Verification items for the finished model (mm, model axes). Coordinates: 2 decimals unless noted, no trailing zeros. Order: outer loops, then holes, each group sorted by start corner. A loop starts at its lowest first (then second) coordinate and runs counter-clockwise, first axis right, second up. Notation, with made-up numbers: M 77,69 L 128,69 A13 cw 128,93 Z; hole C 10.5,53.25 d7. An arc over 180 degrees is marked long. Write item = value, one per line.
```python
from build123d import *

# Parameters (mm, degrees)
SKETCH1_W      = 9.525
SKETCH1_H      = 24.13
EXTRUDE1_DEPTH = 9.525
SKETCH2_R      = 1.5875
EXTRUDE2_DEPTH = 10.525
EXTRUDE3_DEPTH = 9.525


with BuildPart() as part:
    # Sketch1 → Extrude1 (new body)
    with BuildSketch(Plane(origin=(0, 0, 0), x_dir=(1, 0, 0), z_dir=(0, 1, 0))):
        Rectangle(SKETCH1_W, SKETCH1_H)
    extrude(amount=EXTRUDE1_DEPTH)

    # Sketch2 → Extrude2 (cut, through all)
    with BuildSketch(Plane(origin=(4.7625, 0, 0), x_dir=(0, 0, -1), z_dir=(1, 0, 0))):
        with Locations((-6.35, 4.7625)):
            Circle(SKETCH2_R)
        with Locations(Location((6.35, 4.7625, 0), (0, 0, 180))):  # turned: the seam where the file's is
            Circle(SKETCH2_R)
    extrude(amount=-EXTRUDE2_DEPTH, mode=Mode.SUBTRACT)

    # Sketch3 → Extrude3 (add, through all)
    with BuildSketch(Plane(origin=(4.7625, 0, 0), x_dir=(0, 0, -1), z_dir=(1, 0, 0))):
        Polygon((-12.065, 9.525), (-18.394320409, 9.525), (-13.074387176, 0.310605347), (-12.065, 0), align=None)
    extrude(amount=-EXTRUDE3_DEPTH)


solid = part.part
```
Item 1: Scan lines: L1, parallel to Y at x = 0, z = 6.35 (3 decimals); L2, parallel to Z at x = -4.5, y = 4.5 (3 decimals); L3, parallel to Y at x = -0.5, z = -7 (3 decimals). Record each from-to range of solid material in increasing order. Write a range as from..to.
Report:
L1 = 0..3.175, 6.35..9.525
L2 = -12.065..-7.916, -4.784..4.784, 7.916..15.493
L3 = 0..3.314, 6.211..9.525
Item 2: Sectioned sample at B-B, the plane x = 0.5. Give the number of separate pieces and of enclosed holes in the cut face, then the cut area to 3 significant figures.
Report:
separate_pieces = 1
enclosed_holes = 2
area = 248 mm^2
Item 3: Release check for a two-part mould opening along Z. For faces 1 (the cylindrical face through (0.067, 4.286, -4.836)), 2 (the flat face through (0.07, 0.16, 12.58)), 3 (the cylindrical face through (0.067, 6.101, 5.497)), 4 (the flat face through (0, 0, 0)) record: pulls with the +Z half, pulls with the -Z half, needs draft (parallel to the pull), parting line crosses it, or undercut.
Report:
face_1 = undercut
face_2 = pulls with the +Z half
face_3 = undercut
face_4 = needs draft
Item 4: Sectioned sample at C-C, the plane z = 16.5. Enter the section's corners in (x, y) (1 decimal).
Report:
outline = M -4.8,6.2 L 4.8,6.2 L 4.8,9.5 L -4.8,9.5 Z
Item 5: Gauge pin test, flat end, axial feed: pin 1 (4 mm diameter, centred on x = 2, z = 14.5, fed in from -Y). Record the tip position at first contact, or that the pin passes through.
Report:
pin_1 = 0.13
